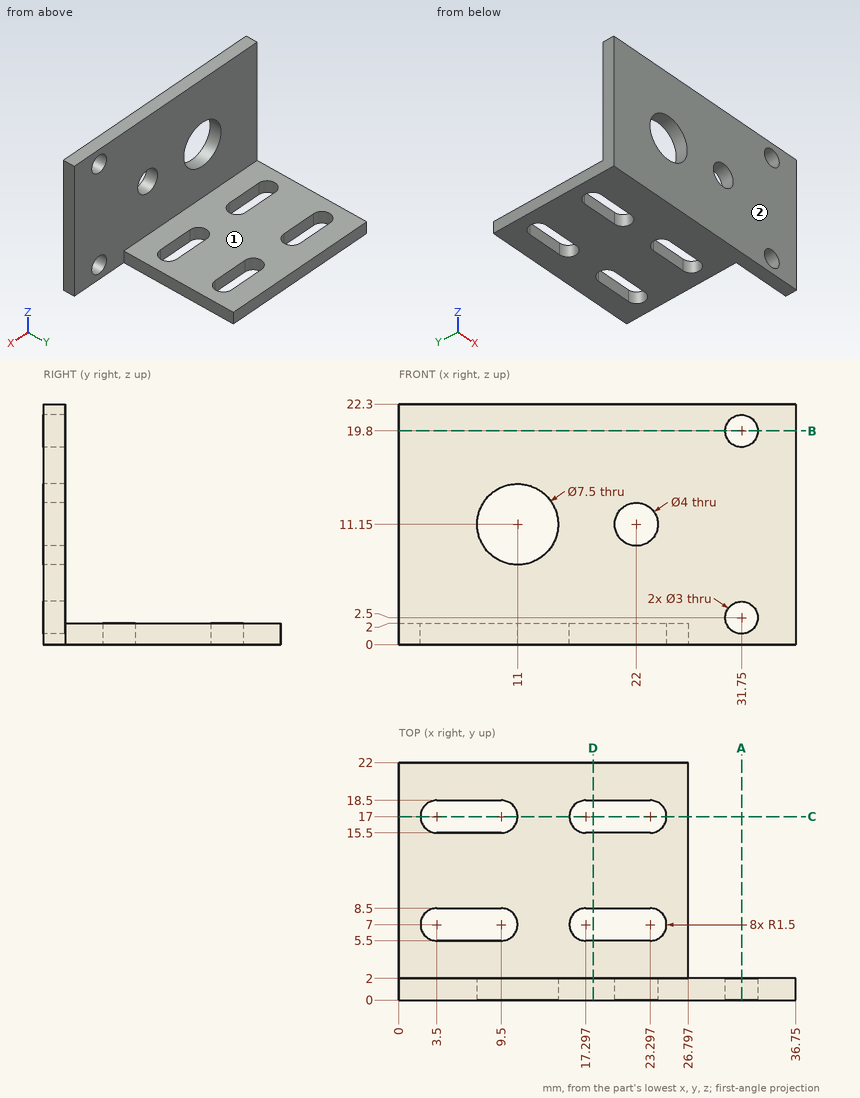
Answer from the drawing. Dimensions are ordinates in mm from the lowest x, y and z of the part. A direction names the side the tool comes from. Give positions to 0.01 mm unless a question says otherwise; leave off trailing zeros. Write each loop counter-clockwise with the first axis right and the second up, starting at its lowest first coordinate (ties: lowest second). Pieces come first, ordered by that corner, then holes. Notation, with made-up numbers: (81, 42.5) - (119, 42.5) arc R27 ccw to (119, 77.5) - close; hole circle Ø10 at (63.25, 70.25). An arc over 180 degrees is marked (long way). Answer in a Markdown table with one row per item. Add a question column.
Item 1: Find the intervals of material crossed by L1, parallel to Z at x = 31.75, y = 0.55; L2, parallel to Z at x = 11, y = 1.3; L3, parallel to Z at x = 22, y = 1.45, in increasing order.
Item 2: Flat-ended cylindrical pins translate along their axes: P1, Ø2, axis at x = 12, z = 13.5, coming from the -Y side; P2, Ø1.6, axis at y = 12.5, z = 0.5, coming from the +X side; P3, Ø2, axis at x = 8.5, y = 14.5, coming from the +Z side; P4, Ø6.5, axis at x = 19.5, z = 14.5, coming from the +Y side. Find the tip coordinate at first contact, or state that the pin passes through.
Item 3: Section A-A, the plane x = 31.75 is taken. Write down the section's boundary in (y, z).
Item 4: Section D-D, the plane x = 18 is taken. Write down the section's boundary in (y, z).
Item 5: A tool of negligible diameter and unlimited length cuts with its end or side. For the marked faces 1 and 2, from which of +Z, -Z, +X, -X, +Y, -Y can it reach the whole face along a straight path? Write none if from no direction.
Item 6: Section C-C, the plane y = 17 is taken. Write down the section's boundary in (x, z).
Item 7: Section B-B, the plane z = 19.8 is taken. Write down the section's boundary in (x, y).
Recorded:
| question | item | result |
|---|---|---|
| 1 | L1 | z = 0 to 1, 4 to 18.3, 21.3 to 22.3 |
| 1 | L2 | z = 0 to 7.4, 14.9 to 22.3 |
| 1 | L3 | z = 0 to 9.15, 13.15 to 22.3 |
| 2 | P1 | passes through |
| 2 | P2 | stops at x = 26.8 |
| 2 | P3 | stops at z = 2 |
| 2 | P4 | stops at y = 2 |
| 3 | outline | (0, 0) - (2, 0) - (2, 1) - (0, 1) - close; (0, 4) - (2, 4) - (2, 18.3) - (0, 18.3) - close; (0, 21.3) - (2, 21.3) - (2, 22.3) - (0, 22.3) - close |
| 4 | outline | (0, 0) - (5.5, 0) - (5.5, 2) - (2, 2) - (2, 22.3) - (0, 22.3) - close; (8.5, 0) - (15.5, 0) - (15.5, 2) - (8.5, 2) - close; (18.5, 0) - (22, 0) - (22, 2) - (18.5, 2) - close |
| 5 | face 1 | +Z, +X, -X, +Y |
| 5 | face 2 | +Z, -Z, +X, -X, -Y |
| 6 | outline | (0, 0) - (2, 0) - (2, 2) - (0, 2) - close; (11, 0) - (15.8, 0) - (15.8, 2) - (11, 2) - close; (24.8, 0) - (26.8, 0) - (26.8, 2) - (24.8, 2) - close |
| 7 | outline | (0, 0) - (30.25, 0) - (30.25, 2) - (0, 2) - close; (33.25, 0) - (36.75, 0) - (36.75, 2) - (33.25, 2) - close |
